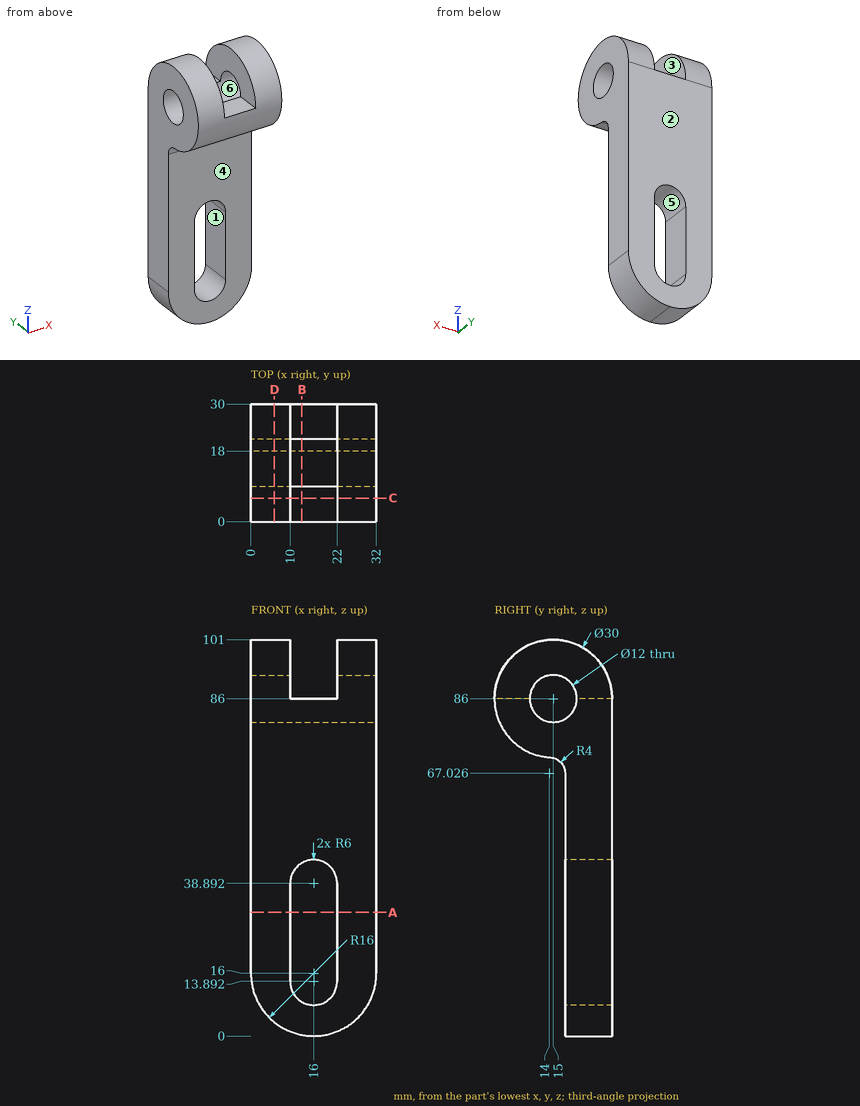
Check sheet for the drawn part. Datum: minimum x, y, z corner. Units: mm. A direction names the side the tool comes from. Give positions to 0.01 mm unless a question says otherwise; leave off trailing zeros. Order: outer loops, then holes, each group sorted by start corner. A loop starts at its lowest first (then second) coordinate and runs counter-clockwise, first axis right, second up. Notation, with made-up numbers: (-20, -29.5) -> (28, -29.5) arc R10 ccw to (28, -21.5) -> close; hole circle Ø3 at (64, -1.75). An arc over 180 degrees is marked (long way). Use a Markdown table: item, result.
1) Section check C-C, the plane y = 6. Record the boundary of the cut face in (x, z).
Results:
| item | result |
|---|---|
| outline | (0, 74) -> (32, 74) -> (32, 98) -> (22, 98) -> (22, 86) -> (10, 86) -> (10, 98) -> (0, 98) -> close |
2) Tool access check on the marked faces 1, 2 and 3. Record the directions out of +Z, -Z, +X, -X, +Y, -Y that give a thin tool (end or side, any length) a straight path to the whole face; none if there is none.
Results:
| item | result |
|---|---|
| face 1 | +Y, -Y |
| face 2 | +Z, -Z, +X, -X, +Y |
| face 3 | +Z, +Y, -Y |
3) Mould release check, pull along Y, two halves, no side actions. Record for the marked faces 4, 5 and 6: pulls with the +Y half, pulls with the -Y half, needs draft (parallel to the pull), parting line crosses it, or undercut.
Results:
| item | result |
|---|---|
| face 4 | pulls with the -Y half |
| face 5 | needs draft |
| face 6 | undercut |
4) Section check D-D, the plane x = 6. Record the boundary of the cut face in (y, z), then the cut area to 3 significant figures.
Results:
| item | result |
|---|---|
| outline | (14.21, 71.02) arc R4 cw to (18, 67.03) -> (18, 3.51) -> (30, 3.51) -> (30, 86) arc R15 ccw (long way) to start; hole circle Ø12 at (15, 86) |
| area | 1,460 mm² |
5) Section check B-B, the plane x = 13. Record the boundary of the cut face in (y, z).
Results:
| item | result |
|---|---|
| outline | (0, 86) arc R15 ccw to (14.21, 71.02) arc R4 cw to (18, 67.03) -> (18, 44.09) -> (30, 44.09) -> (30, 86) -> (21, 86) arc R6 cw to (9, 86) -> close; (18, 0.28) -> (30, 0.28) -> (30, 8.7) -> (18, 8.7) -> close |
6) Depth check by flat-ended pin: pin 1 Ø1 at (y, z) = (24.5, 13) entering from +X; pin 2 Ø7 at (x, y) = (17, 6.5) entering from +Z; pin 3 Ø1.5 at (x, y) = (18, 18) entering from -Z; pin 4 Ø4.5 at (y, z) = (17, 94) entering from -X. Enter the tip coordinate at first touch or a pass-through.
Results:
| item | result |
|---|---|
| pin 1 | x = 31.8 |
| pin 2 | z = 86 |
| pin 3 | z = 0.05 |
| pin 4 | x = 0 |
7) Material ranges on probe 1 along X at (y, z) = (25, 24); probe 2 along Y at (x, z) = (7.5, 86); probe 3 along Y at (x, z) = (1.5, 20), recorded low to high.
Results:
| item | result |
|---|---|
| probe 1 | 0 to 10, 22 to 32 |
| probe 2 | 0 to 9, 21 to 30 |
| probe 3 | 18 to 30 |
8) Section check A-A, the plane z = 31.5. Record the boundary of the cut face in (x, y).
Results:
| item | result |
|---|---|
| outline | (0, 18) -> (10, 18) -> (10, 30) -> (0, 30) -> close; (22, 18) -> (32, 18) -> (32, 30) -> (22, 30) -> close |
